from build123d import *

# Parameters (mm, degrees)
SKETCH_1_W           = 37.5
SKETCH_1_H           = 54
EXTRUDE_1_DEPTH      = 3
EXTRUDE_2_DEPTH      = 19.9
EXTRUDE_2_DEPTH_BACK = 3
SKETCH_2_W           = 6
SKETCH_2_H           = 7.6
SKETCH_3_R           = 1.75
CUT_EXTRUDE_1_DEPTH  = 42.775830333
SKETCH_4_R           = 1.75
CUT_EXTRUDE_2_DEPTH  = 40.135310143


with BuildPart() as part:
    # 草图1 → 凸台-拉伸1 (new body)
    with BuildSketch(Plane(origin=(0, 0, 0), x_dir=(1, 0, 0), z_dir=(0, 1, 0))):
        Rectangle(SKETCH_1_W, SKETCH_1_H)
    extrude(amount=EXTRUDE_1_DEPTH)

    # 草图2 → 凸台-拉伸2 (add, two sides: drawn at the far end of the back side and taken through both)
    with BuildSketch(Plane(origin=(0, 3, 0), x_dir=(1, 0, 0), z_dir=(0, 1, 0)).offset(-EXTRUDE_2_DEPTH_BACK)):
        with Locations((-5.15, -24.2)):
            Rectangle(SKETCH_2_W, SKETCH_2_H)
        with Locations((-5.15, 24.2)):
            Rectangle(SKETCH_2_W, SKETCH_2_H)
    extrude(amount=EXTRUDE_2_DEPTH + EXTRUDE_2_DEPTH_BACK)

    # 草图3 → 切除-拉伸1 (cut, through all)
    with BuildSketch(Plane(origin=(-2.15, 0, 0), x_dir=(0, 0, -1), z_dir=(1, 0, 0))):
        with Locations((-24.3, 17.9)):
            Circle(SKETCH_3_R)
        with Locations((-24.3, 8)):
            Circle(SKETCH_3_R)
        with Locations((24.3, 8)):
            Circle(SKETCH_3_R)
        with Locations((24.3, 17.9)):
            Circle(SKETCH_3_R)
    extrude(amount=-CUT_EXTRUDE_1_DEPTH, mode=Mode.SUBTRACT)

    # 草图4 → 切除-拉伸2 (cut, through all)
    with BuildSketch(Plane(origin=(0, 3, 0), x_dir=(1, 0, 0), z_dir=(0, 1, 0))):
        with Locations(Location((-15.75, 24, 0), (0, 0, 270))):
            Circle(SKETCH_4_R)
        with Locations(Location((-15.75, -24, 0), (0, 0, 270))):
            Circle(SKETCH_4_R)
        with Locations(Location((15.75, -24, 0), (0, 0, 270))):
            Circle(SKETCH_4_R)
        with Locations(Location((15.75, 24, 0), (0, 0, 270))):
            Circle(SKETCH_4_R)
    extrude(amount=-CUT_EXTRUDE_2_DEPTH, mode=Mode.SUBTRACT)


solid = part.part
Here's how the part is built. I have some questions about the finished solid (model axes, mm). A direction names the side the tool comes from. Give positions to 0.01 mm unless a question says otherwise; leave off trailing zeros. Order: outer loops, then holes, each group sorted by start corner. A loop starts at its lowest first (then second) coordinate and runs counter-clockwise, first axis right, second up. Notation, with made-up numbers: M 37.25,88.5 L 51.25,88.5 A20 ccw 51.25,92.5 Z; hole C -13.75,3.5 d2. An arc over 180 degrees is marked long. Answer as a JSON object with one key per item and string values. Group by question number.
1) Suppose I cut it at A-A, the plane y = 15.5. Write out the boundary of the cut face in (x, z), plus the area to 3 significant figures.
2) Suppose I cut it at C-C, the plane y = 8. Write out the boundary of the cut face in (x, z).
3) We'd pull the mould along Z, two halves only. Please class faces 6 (the flat face through (-5, 11, -28)), 7 (the cylindrical face through (-5.11, 16.35, -25.11)), 8 (the flat face through (-8.15, 11, -24)): pulls with the +Z half, pulls with the -Z half, needs draft (parallel to the pull), parting line crosses it, or undercut.
4) On a 3-axis mill with a long thin cutter (end or side, diameter ignored), from which of +Z, -Z, +X, -X, +Y, -Y can I reach the whole of each face in a straight line? I mean faces 1 (the flat face through (-5, 13, -20.4)), 2 (the flat face through (8, 1, 27)), 3 (the flat face through (-14, 1, -27)), 4 (the flat face through (8, 1, -27)), 5 (the flat face through (-14, 1, 27)). Say none if no direction works.
5) I'm going to push flat-ended pins straight in: pin 1 Ø2 at (x, z) = (-12.5, -13.5) entering from +Y; pin 2 Ø3.5 at (x, y) = (11, 1) entering from -Z; pin 3 Ø2 at (x, z) = (-15, -5.5) entering from -Y; pin 4 Ø4.5 at (y, z) = (17.9, 24.3) entering from +X. Where does each tip first touch, or does it pass through?
6) Suppose I cut it at B-B, the plane x = 15.75. Write out the boundary of the cut face in (y, z).
7) Please list where these lines run through material, in increasing order: L1, parallel to Y at x = -3.95, z = 24.3; L2, parallel to X at y = 0.85, z = -24; L3, parallel to Z at x = -3.5, y = 10.5. Write a range as [from, to].
8) Suppose I cut it at D-D, the plane z = 24.3. Write out the boundary of the cut face in (x, y), plus the area to 3 significant figures.
Results found:
{
 "1": {"outline": "M -8.15,-28 L -2.15,-28 L -2.15,-20.4 L -8.15,-20.4 Z; M -8.15,20.4 L -2.15,20.4 L -2.15,28 L -8.15,28 Z", "area": "91.2 mm²"},
 "2": {"outline": "M -8.15,-28 L -2.15,-28 L -2.15,-26.05 L -8.15,-26.05 Z; M -8.15,-22.55 L -2.15,-22.55 L -2.15,-20.4 L -8.15,-20.4 Z; M -8.15,20.4 L -2.15,20.4 L -2.15,22.55 L -8.15,22.55 Z; M -8.15,26.05 L -2.15,26.05 L -2.15,28 L -8.15,28 Z"},
 "3": {"face 6": "pulls with the -Z half", "face 7": "undercut", "face 8": "needs draft"},
 "4": {"face 1": "+X, -X, +Y", "face 2": "+Z, +X, +Y, -Y", "face 3": "-Z, -X, +Y, -Y", "face 4": "-Z, +X, +Y, -Y", "face 5": "+Z, -X, +Y, -Y"},
 "5": {"pin 1": "y = 3", "pin 2": "z = -27", "pin 3": "y = 0", "pin 4": "x = -2.15"},
 "6": {"outline": "M 0,-27 L 3,-27 L 3,-25.75 L 0,-25.75 Z; M 0,-22.25 L 3,-22.25 L 3,22.25 L 0,22.25 Z; M 0,25.75 L 3,25.75 L 3,27 L 0,27 Z"},
 "7": {"L1": "[0, 6.25], [9.75, 16.15], [19.65, 22.9]", "L2": "[-18.75, -17.5], [-14, 14], [17.5, 18.75]", "L3": "[-28, -20.4], [20.4, 28]"},
 "8": {"outline": "M -18.75,0 L -17.47,0 L -17.47,3 L -18.75,3 Z; M -14.03,0 L 14.03,0 L 14.03,3 L -2.15,3 L -2.15,6.25 L -8.15,6.25 L -8.15,3 L -14.03,3 Z; M -8.15,9.75 L -2.15,9.75 L -2.15,16.15 L -8.15,16.15 Z; M -8.15,19.65 L -2.15,19.65 L -2.15,22.9 L -8.15,22.9 Z; M 17.47,0 L 18.75,0 L 18.75,3 L 17.47,3 Z", "area": "169 mm²"}
}
